Can you work these out from the drawing? Everything is in mm from the part's minimum corner. A direction names the side the tool comes from. Give positions to 0.01 mm unless a question says otherwise; leave off trailing zeros. Write each loop counter-clockwise with the first axis right and the second up, starting at its lowest first coordinate (ties: lowest second). Pieces come first, ordered by that corner, then holes. Notation, with made-up numbers: (51, 3) - (109, 3) arc R23 ccw to (109, 38) - close; hole circle Ø11 at (42.25, 53). An arc over 180 degrees is marked (long way). Use a Markdown table: item, result. Add a question column.
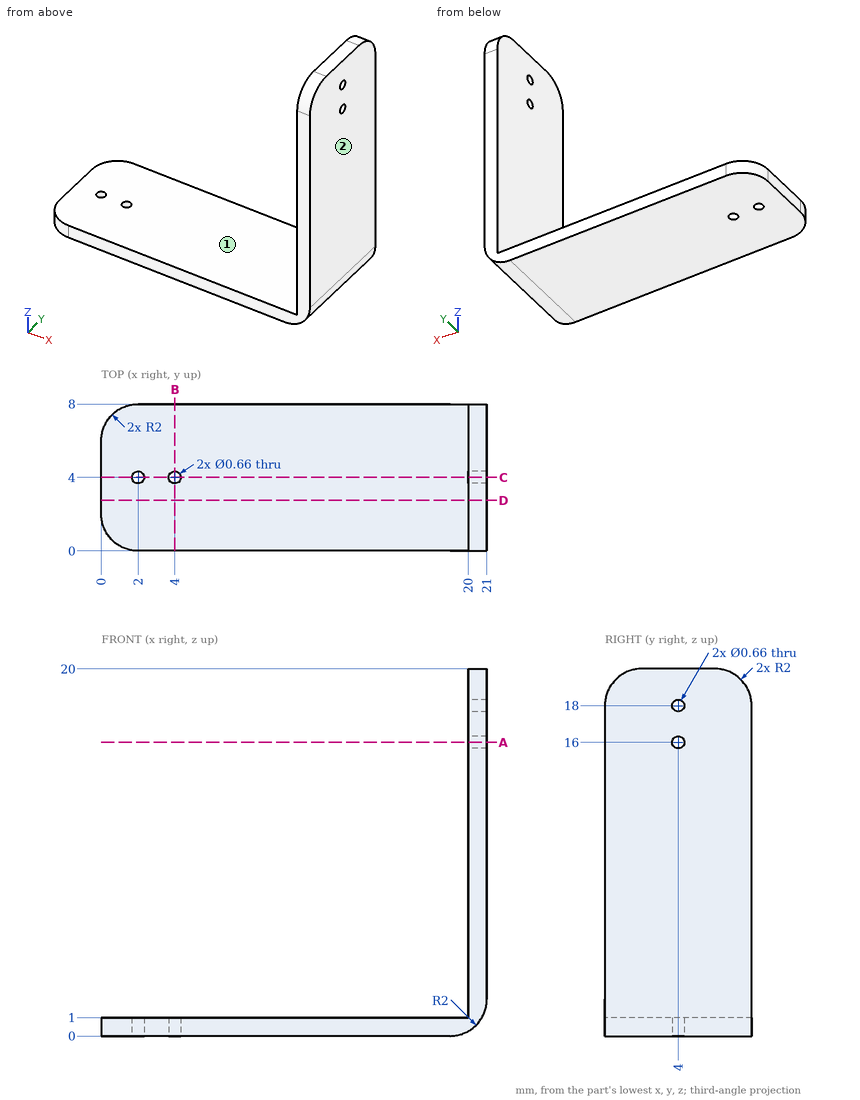
Q1. Suppose I cut it at D-D (y = 2.75). Please give me the cut outline in (x, z).
Q2. Suppose I cut it at C-C (y = 4). Please give me the cut outline in (x, z).
Q3. Suppose I cut it at A-A (z = 16). Please give me the cut outline in (x, y).
Q4. If I drill on probe 1 along Y at (x, z) = (20.6, 18); probe 2 along Z at (x, y) = (7.75, 3.5); probe 3 along X at (y, z) = (4.5, 18.25), over which ranges is the centre line in solid material (lowest first)? Write a range as [from, to].
Q5. I'm going to push flat-ended pins straight in: P1, Ø4, axis at x = 4, y = 2.5, coming from the +Z side; P2, Ø3, axis at x = 6, z = 4, coming from the +Y side. Where does each tip first touch, or does it pass through?
Q6. On a 3-axis mill with a long thin cutter (end or side, diameter ignored), from which of +Z, -Z, +X, -X, +Y, -Y can I reach the whole of each face in a straight line? I mean the marked faces 1 and 2. Say none if no direction works.
Q7. Suppose I cut it at B-B (x = 4). Please give me the cut outline in (y, z).
Derived:
| question | item | result |
|---|---|---|
| 1 | outline | (0, 0) - (19, 0) arc R2 ccw to (21, 2) - (21, 20) - (20, 20) - (20, 1) - (0, 1) - close |
| 2 | outline | (0, 0) - (1.67, 0) - (1.67, 1) - (0, 1) - close; (2.33, 0) - (3.67, 0) - (3.67, 1) - (2.33, 1) - close; (4.33, 0) - (19, 0) arc R2 ccw to (21, 2) - (21, 15.67) - (20, 15.67) - (20, 1) - (4.33, 1) - close; (20, 16.33) - (21, 16.33) - (21, 17.67) - (20, 17.67) - close; (20, 18.33) - (21, 18.33) - (21, 20) - (20, 20) - close |
| 3 | outline | (20, 0) - (21, 0) - (21, 3.67) - (20, 3.67) - close; (20, 4.33) - (21, 4.33) - (21, 8) - (20, 8) - close |
| 4 | probe 1 | [0, 3.67], [4.33, 8] |
| 4 | probe 2 | [0, 1] |
| 4 | probe 3 | [20, 21] |
| 5 | P1 | z = 1 |
| 5 | P2 | through |
| 6 | face 1 | +Z, -X, +Y, -Y |
| 6 | face 2 | +Z, -Z, +X, +Y, -Y |
| 7 | outline | (0, 0) - (3.67, 0) - (3.67, 1) - (0, 1) - close; (4.33, 0) - (8, 0) - (8, 1) - (4.33, 1) - close |
